Work out the finished part from the listing and answer in its coordinate system (mm). A direction names the side the tool comes from. Round coordinates to 2 decimals unless told otherwise and drop trailing zeros. Write each loop counter-clockwise with the first axis right and the second up, starting at its lowest first coordinate (ties: lowest second). Pieces come first, ordered by that corner, then holes. Notation, with made-up numbers: (33.25, 26) - (90.25, 26) arc R19 cw to (90.25, 32) - close; hole circle Ø5 at (-7.5, 41.5). An arc over 180 degrees is marked (long way). Answer as a JSON object with one key per item and string values.
```python
from build123d import *

# Parameters (mm, degrees)
CUT_EXTRUDE1_DEPTH = 2


with BuildPart() as part:
    # Sketch1 → Revolve1 (revolve)
    with BuildSketch(Plane.XY, mode=Mode.PRIVATE) as revolve1_sk:
        Polygon((0.9, -2), (0.9, 2), (0, 2), (0, 5), (20, 5), (20, 2), (2.9, 2), (2.9, -2), align=None)
    revolve(revolve1_sk.sketch.rotate(Axis((0, -3.539189189, 0), (0, 1, 0)), 90), axis=Axis((0, -3.539189189, 0), (0, 1, 0)))

    # Sketch2 → Cut-Extrude1 (cut)
    with BuildSketch(Plane(origin=(0, 5, 0), x_dir=(1, 0, 0), z_dir=(0, 1, 0))):
        with BuildLine():
            Line((0.526272079, 19.119202876), (-9.2795165, 10.133853114))
            ThreePointArc((-9.2795165, 10.133853114), (-5.338676553, 0), (-9.2795165, -10.133853114))
            Line((-9.2795165, -10.133853114), (0.526272079, -19.119202876))
            ThreePointArc((0.526272079, -19.119202876), (7.961323447, 0), (0.526272079, 19.119202876))
        make_face()
    extrude(amount=-CUT_EXTRUDE1_DEPTH, mode=Mode.SUBTRACT)


solid = part.part
```
Item 1: Each of these flat-tipped pins is pushed along its axis until it touches: P1, Ø1.5, axis at y = 4, z = -12, coming from the +X side; P2, Ø1, axis at x = 1, y = -1, coming from the -Z side; P3, Ø1.5, axis at x = 15.5, z = 9.5, coming from the -Y side. Where does it stop, or does it pass through?
Results found:
{"P1": "x = 16.54", "P2": "z = -2.86", "P3": "y = 2"}
Item 2: A cutting plane is placed at D-D (z = 17). Write down the section's boundary in (x, y), and give its area (3 significant figures).
Results found:
{"outline": "(-10.54, 2) - (10.54, 2) - (10.54, 5) - (2.29, 5) - (2.29, 3) - (-1.79, 3) - (-1.79, 5) - (-10.54, 5) - close", "area": "55.1 mm²"}
Item 3: For faces 5 (the flat face through (0, 2, 0)), 6 (the flat face through (9, 5, 0)), 7 (the cylindrical face through (7.96, 4.01, 0.29)), determine the directions among +Z, -Z, +X, -X, +Y, -Y from which every point of the face is accessible in a straight line to the end or side of a thin tool.
Results found:
{"face 5": "-Y", "face 6": "+Z, -Z, +X, -X, +Y", "face 7": "+Y"}
Item 4: Consider line 1 along X through (y, z) = (-0.75, 0); line 2 along Y through (x, z) = (5.5, -11); line 3 along Y through (x, z) = (9, 11.5). Determine where each line is inside the solid, lowest interval first.
Results found:
{"line 1": "-2.9 to -0.9, 0.9 to 2.9", "line 2": "2 to 3", "line 3": "2 to 5"}
Item 5: A cutting plane is placed at B-B (z = 0). Write down the section's boundary in (x, y), and give its area (3 significant figures).
Results found:
{"outline": "(-20, 2) - (-2.9, 2) - (-2.9, -2) - (-0.9, -2) - (-0.9, 2) - (0.9, 2) - (0.9, -2) - (2.9, -2) - (2.9, 2) - (20, 2) - (20, 5) - (7.96, 5) - (7.96, 3) - (-5.34, 3) - (-5.34, 5) - (-20, 5) - close", "area": "109 mm²"}
Item 6: Determine the mould class of faces 1 (the flat face through (-4.45, 4.01, 14.56)), 2 (the cylindrical face through (-0.88, 3.48, 19.98)), 3 (the flat face through (-1, -2, -1)), 4 (the cylindrical face through (-0.27, 0.03, -0.86)) for opening direction X: pulls with the +X half, pulls with the -X half, needs draft (parallel to the pull), parting line crosses it, or undercut.
Results found:
{"face 1": "undercut", "face 2": "parting line crosses it", "face 3": "needs draft", "face 4": "undercut"}
Item 7: A cutting plane is placed at C-C (x = 6). Write down the section's boundary in (y, z).
Results found:
{"outline": "(2, -19.08) - (5, -19.08) - (5, -10.35) - (3, -10.35) - (3, 10.35) - (5, 10.35) - (5, 19.08) - (2, 19.08) - close"}
Item 8: A cutting plane is placed at A-A (y = 4.5). Write down the section's boundary in (x, z).
Results found:
{"outline": "circle Ø40 at (0, 0); hole (-9.28, -10.13) - (0.53, -19.12) arc R28.3 ccw to (0.53, 19.12) - (-9.28, 10.13) arc R15 cw to start"}
